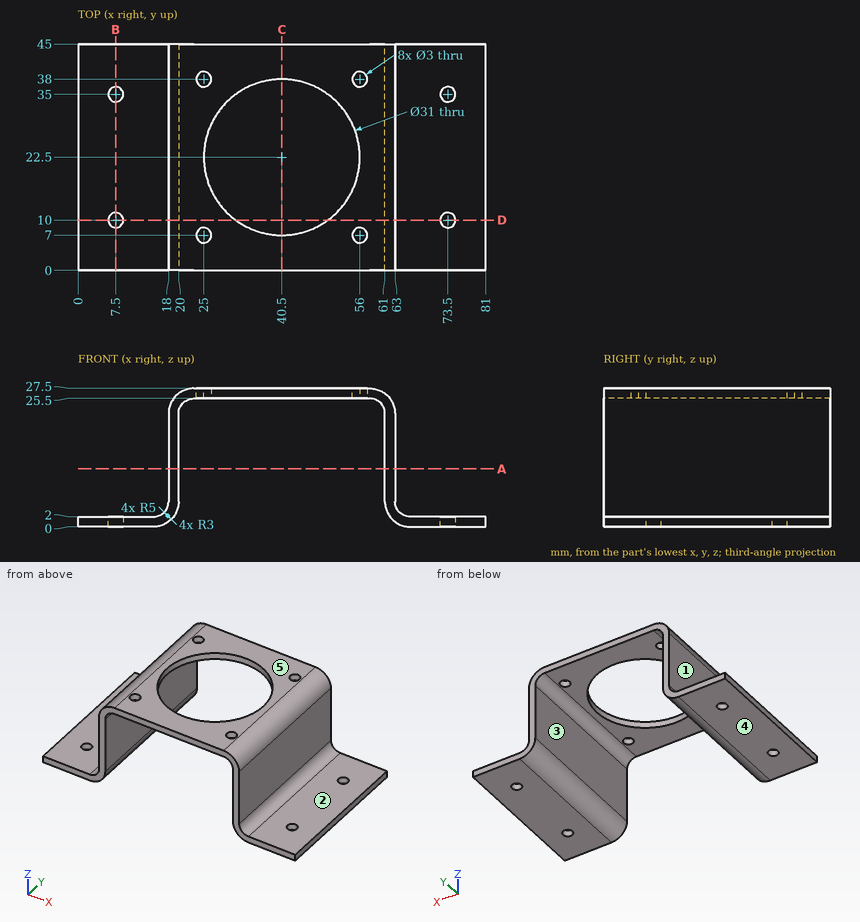
Could you check a few things on this drawing? It's one solid part, dimensions in mm from its lowest x, y, z. A direction names the side the tool comes from. Coordinates: 2 decimals unless noted, no trailing zeros. Order: outer loops, then holes, each group sorted by start corner. A loop starts at its lowest first (then second) coordinate and runs counter-clockwise, first axis right, second up. Notation, with made-up numbers: M 52.5,64 L 67.5,64 A24 cw 67.5,78 Z; hole C -22,-33.75 d6. An arc over 180 degrees is marked long. Use one line per item in the form item = value. Start each with the question number.
1. Suppose I cut it at B-B on x = 7.5. Write out the boundary of the cut face in (y, z).
2. Please list where these lines run through material, in increasing order: line 1 (Y direction, x = 7.5, z = 1.6); line 2 (X direction, y = 36, z = 6.25); line 3 (Z direction, x = 74, y = 26).
3. On a 3-axis mill with a long thin cutter (end or side, diameter ignored), from which of +Z, -Z, +X, -X, +Y, -Y can I reach the whole of each face in a straight line? I mean the marked faces 1, 2, 3, 4 and 5. Say none if no direction works.
4. Suppose I cut it at C-C on x = 40.5. Write out the boundary of the cut face in (y, z), then the cut area to 3 significant figures.
5. Suppose I cut it at D-D on y = 10. Count the separate pieces of the cut face and the enclosed holes in it, then the cut area to 3 significant figures.
6. Suppose I cut it at A-A on z = 11.5. Write out the boundary of the cut face in (x, y).
7. For pin 1 (10 mm diameter, centred on x = 57.5, z = 8, fed in from +Y); pin 2 (2 mm diameter, centred on y = 27, z = 18, fed in from +X); pin 3 (16.5 mm diameter, centred on x = 5.5, y = 17, fed in from +Z); pin 4 (3.5 mm diameter, centred on x = 25, y = 38, fed in from -Z), each with a flat end and sliding along its axis, tell me the tip position at first contact or that it passes through.
Geometry says:
q1.outline = M 0,0 L 8.5,0 L 8.5,2 L 0,2 Z; M 11.5,0 L 33.5,0 L 33.5,2 L 11.5,2 Z; M 36.5,0 L 45,0 L 45,2 L 36.5,2 Z
q2.line_1 = 0 to 8.5, 11.5 to 33.5, 36.5 to 45
q2.line_2 = 18 to 20, 61 to 63
q2.line_3 = 0 to 2
q3.face_1 = +Z, -X, +Y, -Y
q3.face_2 = +Z, +X, +Y, -Y
q3.face_3 = -Z, +Y, -Y
q3.face_4 = -Z, +X, -X, +Y, -Y
q3.face_5 = +Z, +X, -X, +Y, -Y
q4.outline = M 0,25.5 L 7,25.5 L 7,27.5 L 0,27.5 Z; M 38,25.5 L 45,25.5 L 45,27.5 L 38,27.5 Z
q4.area = 28.0 mm^2
q5.separate_pieces = 4
q5.enclosed_holes = 0
q5.area = 202 mm^2
q6.outline = M 18,0 L 20,0 L 20,45 L 18,45 Z; M 61,0 L 63,0 L 63,45 L 61,45 Z
q7.pin_1 = 45
q7.pin_2 = 63
q7.pin_3 = 2
q7.pin_4 = 25.5
